Part print with two shaded views. Sizes in mm from the minimum x, y, z corner. Coordinates: 2 decimals unless noted, no trailing zeros. Order: outer loops, then holes, each group sorted by start corner. A loop starts at its lowest first (then second) coordinate and runs counter-clockwise, first axis right, second up.
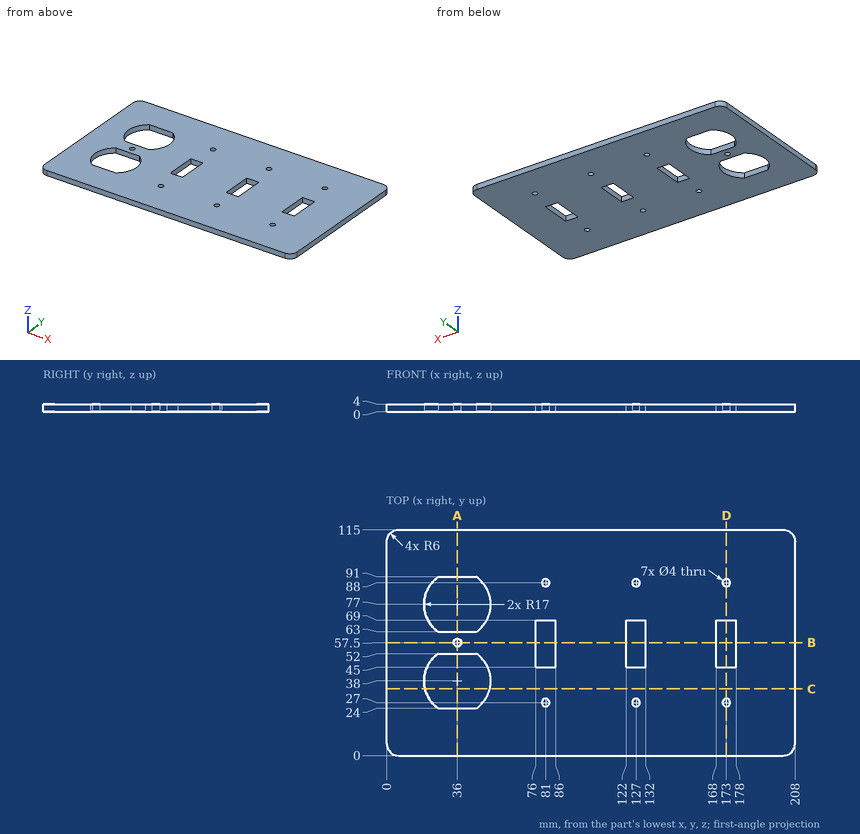
Q1. Pin check, flat tip, straight feed: pin 1 Ø2.5 at (x, y) = (81, 88) entering from +Z. Stop position of the tip, or through.
Results list:
pin 1: passes through
Q2. Cut at B-B on y = 57.5. Write the cut outline in (x, z).
Results list:
outline: (0, 0) - (34, 0) - (34, 4) - (0, 4) - close; (38, 0) - (76, 0) - (76, 4) - (38, 4) - close; (86, 0) - (122, 0) - (122, 4) - (86, 4) - close; (132, 0) - (168, 0) - (168, 4) - (132, 4) - close; (178, 0) - (208, 0) - (208, 4) - (178, 4) - close
Q3. Wall check: line 1 along Y through (x, z) = (127, 2.2); line 2 along Y through (x, z) = (43, 1.4); line 3 along X through (y, z) = (49, 2.05). Give the ranges that are in metal, low to high.
Results list:
line 1: y = 0 to 25, 29 to 45, 69 to 86, 90 to 115
line 2: y = 0 to 24, 52 to 63, 91 to 115
line 3: x = 0 to 23.04, 48.96 to 76, 86 to 122, 132 to 168, 178 to 208
Q4. Cut at D-D on x = 173. Write the cut outline in (y, z), and give its area (3 significant figures).
Results list:
outline: (0, 0) - (25, 0) - (25, 4) - (0, 4) - close; (29, 0) - (45, 0) - (45, 4) - (29, 4) - close; (69, 0) - (86, 0) - (86, 4) - (69, 4) - close; (90, 0) - (115, 0) - (115, 4) - (90, 4) - close
area: 332 mm2
Q5. Cut at A-A on x = 36. Write the cut outline in (y, z), and give its area (3 significant figures).
Results list:
outline: (0, 0) - (24, 0) - (24, 4) - (0, 4) - close; (52, 0) - (55.5, 0) - (55.5, 4) - (52, 4) - close; (59.5, 0) - (63, 0) - (63, 4) - (59.5, 4) - close; (91, 0) - (115, 0) - (115, 4) - (91, 4) - close
area: 220 mm2
Q6. Cut at C-C on y = 34. Write the cut outline in (x, z).
Results list:
outline: (0, 0) - (19.48, 0) - (19.48, 4) - (0, 4) - close; (52.52, 0) - (208, 0) - (208, 4) - (52.52, 4) - close
